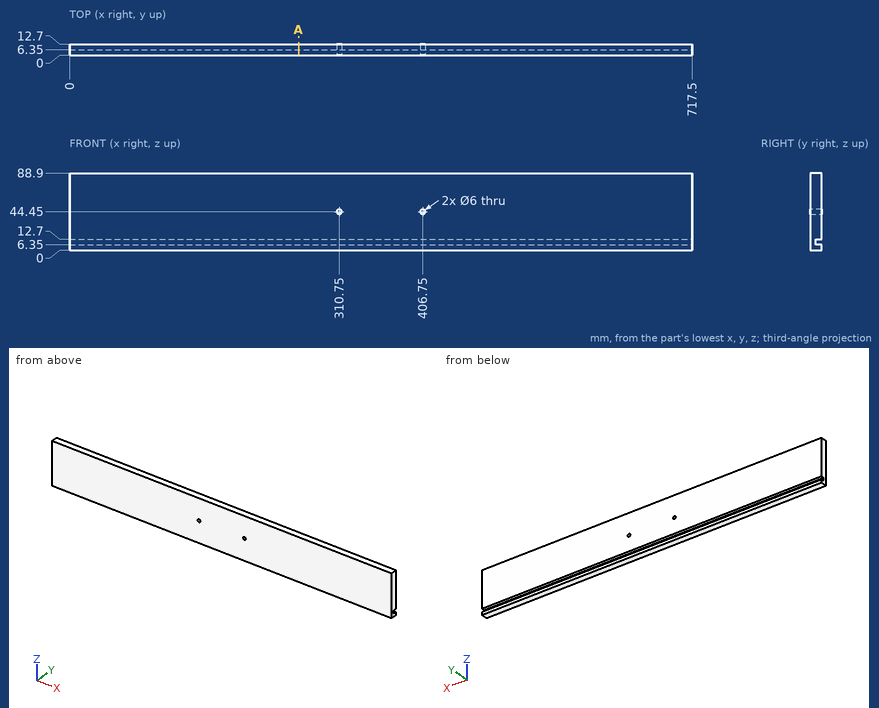
Answer from the drawing. Dimensions are ordinates in mm from the lowest x, y and z of the part. Give positions to 0.01 mm unless a question says otherwise; leave off trailing zeros. Order: outer loops, then holes, each group sorted by start corner. A loop starts at its lowest first (then second) coordinate and runs counter-clockwise, first axis right, second up. Notation, with made-up numbers: (-4, 18.5) - (30, 18.5) arc R21 ccw to (30, 40.5) - close; hole circle Ø8 at (40, 19.5). An arc over 180 degrees is marked (long way). One line per item, written item: value. Start each with the question number.
1. This flat-tipped pin is pushed along its axis until it touches: pin 1 Ø5.5 at (x, z) = (310.75, 44.45) entering from +Y. Where does it stop, or does it pass through?
2. Section A-A, the plane x = 264 is taken. Write down the section's boundary in (y, z), then the cut area to 3 significant figures.
3. Consider line 1 (X direction, y = 4.25, z = 44.45); line 2 (Z direction, x = 310.75, y = 8.75); line 3 (Z direction, x = 280.5, y = 6.75). Determine where each line is inside the solid, lowest interval first.
Filled sheet:
1. pin 1: through
2. outline: (0, 0) - (12.7, 0) - (12.7, 6.35) - (6.35, 6.35) - (6.35, 12.7) - (12.7, 12.7) - (12.7, 88.9) - (0, 88.9) - close
2. area: 1,090 mm²
3. line 1: 0 to 307.75, 313.75 to 403.75, 409.75 to 717.5
3. line 2: 0 to 6.35, 12.7 to 41.45, 47.45 to 88.9
3. line 3: 0 to 6.35, 12.7 to 88.9
